The listing builds one solid part. Answer for the finished solid, in the listing's coordinates (mm). A direction names the side the tool comes from. Coordinates: 2 decimals unless noted, no trailing zeros. Order: outer loops, then holes, each group sorted by start corner. A loop starts at its lowest first (then second) coordinate and runs counter-clockwise, first axis right, second up. Notation, with made-up numbers: (69, 48) -> (122, 48) arc R16 cw to (122, 69) -> close; hole circle Ø8 at (35, 17). An arc over 180 degrees is marked (long way). Answer in a Markdown table with one row per item.
```python
from build123d import *

# Parameters (mm, degrees)
RESSALTO_EXTRUS_O1_DEPTH = 55
ESBO_O2_W                = 15.2
ESBO_O2_H                = 25.2
CORTE_EXTRUS_O1_DEPTH    = 3
ESBO_O4_R                = 1.7
CORTE_EXTRUS_O2_DEPTH    = 31
ESBO_O5_R                = 4.7
CORTE_EXTRUS_O3_DEPTH    = 4
ESBO_O6_R                = 1.75
CORTE_EXTRUS_O4_DEPTH    = 4
ESBO_O7_W                = 15
ESBO_O7_H                = 20
ESBO_O7_R                = 1.65
RESSALTO_EXTRUS_O2_DEPTH = 3


with BuildPart() as part:
    # Esboço1 → Ressalto-extrusão1 (new body)
    with BuildSketch(Plane.XY):
        Polygon((0, 0), (38, 0), (38, 8), (3, 8), (3, 30), (0, 30), align=None)
    extrude(amount=RESSALTO_EXTRUS_O1_DEPTH)

    # Esboço2 → Corte-extrusão1 (cut)
    with BuildSketch(Plane.XZ):
        with Locations((28, 30)):
            Rectangle(ESBO_O2_W, ESBO_O2_H)
    extrude(amount=-CORTE_EXTRUS_O1_DEPTH, mode=Mode.SUBTRACT)

    # Esboço4 → Corte-extrusão2 (cut, through all)
    with BuildSketch(Plane.XZ):
        with Locations((28, 30)):
            Circle(ESBO_O4_R)
        with Locations((28, 10)):
            Circle(ESBO_O4_R)
        with BuildLine():
            Line((29.7, 52.5), (29.7, 49.5))
            ThreePointArc((29.7, 49.5), (28, 47.8), (26.3, 49.5))
            Line((26.3, 49.5), (26.3, 52.5))
            ThreePointArc((26.3, 52.5), (28, 54.2), (29.7, 52.5))
        make_face()
    extrude(amount=-CORTE_EXTRUS_O2_DEPTH, mode=Mode.SUBTRACT)

    # Esboço5 → Corte-extrusão3 (cut)
    with BuildSketch(Plane.XZ):
        with Locations((28, 10)):
            Circle(ESBO_O5_R)
        with BuildLine():
            Line((32.7, 49.5), (32.7, 52.5))
            ThreePointArc((32.7, 52.5), (28, 57.2), (23.3, 52.5))
            Line((23.3, 52.5), (23.3, 49.5))
            ThreePointArc((23.3, 49.5), (28, 44.8), (32.7, 49.5))
        make_face()
    extrude(amount=-CORTE_EXTRUS_O3_DEPTH, mode=Mode.SUBTRACT)

    # Esboço6 → Corte-extrusão4 (cut)
    with BuildSketch(Plane.ZY):
        with Locations((48, 20)):
            Circle(ESBO_O6_R)
        with Locations((3, 20)):
            Circle(ESBO_O6_R)
    extrude(amount=-CORTE_EXTRUS_O4_DEPTH, mode=Mode.SUBTRACT)

    # Esboço7 → Ressalto-extrusão2 (add)
    with BuildSketch(Plane.ZY):
        with Locations((62.5, 10)):
            Rectangle(ESBO_O7_W, ESBO_O7_H)
        with Locations((65, 5.25)):
            Circle(ESBO_O7_R, mode=Mode.SUBTRACT)
        with BuildLine():
            Line((63.35, 13.25), (63.35, 16.25))
            ThreePointArc((63.35, 16.25), (65, 17.9), (66.65, 16.25))
            Line((66.65, 16.25), (66.65, 13.25))
            ThreePointArc((66.65, 13.25), (65, 11.6), (63.35, 13.25))
        make_face(mode=Mode.SUBTRACT)
    extrude(amount=-RESSALTO_EXTRUS_O2_DEPTH)


solid = part.part
```
(1) A cutting plane is placed at C-C, the plane z = 65. Determine the outline of the cut face in (x, y), then the cut area to 3 significant figures.
Check values:
| item | result |
|---|---|
| outline | (0, 0) -> (3, 0) -> (3, 3.6) -> (0, 3.6) -> close; (0, 6.9) -> (3, 6.9) -> (3, 11.6) -> (0, 11.6) -> close; (0, 17.9) -> (3, 17.9) -> (3, 20) -> (0, 20) -> close |
| area | 31.2 mm² |
(2) A cutting plane is placed at B-B, the plane z = 3. Determine the outline of the cut face in (x, y).
Check values:
| item | result |
|---|---|
| outline | (0, 0) -> (38, 0) -> (38, 8) -> (3, 8) -> (3, 18.25) -> (0, 18.25) -> close; (0, 21.75) -> (3, 21.75) -> (3, 30) -> (0, 30) -> close |
(3) Find the intervals of material crossed by line 1 along Z through (x, y) = (28, 4.85); line 2 along Y through (x, z) = (2.25, 3); line 3 along X through (y, z) = (3.5, 7.5), in increasing order. Write a range as from..to.
Check values:
| item | result |
|---|---|
| line 1 | 0..8.3, 11.7..28.3, 31.7..47.8, 54.2..55 |
| line 2 | 0..18.25, 21.75..30 |
| line 3 | 0..24.02, 31.98..38 |
(4) A cutting plane is placed at A-A, the plane y = 5.25. Determine the outline of the cut face in (x, z), then the cut area to 3 significant figures.
Check values:
| item | result |
|---|---|
| outline | (0, 0) -> (38, 0) -> (38, 55) -> (3, 55) -> (3, 63.35) -> (0, 63.35) -> close; (0, 66.65) -> (3, 66.65) -> (3, 70) -> (0, 70) -> close; hole circle Ø3.4 at (28, 10); hole circle Ø3.4 at (28, 30); hole (26.3, 49.5) arc R1.7 ccw to (29.7, 49.5) -> (29.7, 52.5) arc R1.7 ccw to (26.3, 52.5) -> close |
| area | 2,090 mm² |
(5) A cutting plane is placed at D-D, the plane x = 22. Determine the outline of the cut face in (y, z), then the cut area to 3 significant figures.
Check values:
| item | result |
|---|---|
| outline | (0, 0) -> (8, 0) -> (8, 55) -> (0, 55) -> (0, 42.6) -> (3, 42.6) -> (3, 17.4) -> (0, 17.4) -> close |
| area | 364 mm² |
(6) Which of the six approach directions +Z, -Z, +X, -X, +Y, -Y give full straight-line access (tool end or side, diameter ignored) to faces 4 (the flat face through (29.7, 6, 51)), 5 (the flat face through (20, 4, 55)), 6 (the cylindrical face through (1.5, 17.9, 65))?
Check values:
| item | result |
|---|---|
| face 4 | +Y, -Y |
| face 5 | +Z, +X, +Y, -Y |
| face 6 | +X, -X |
(7) For a pull along Y with two mould halves and no side action, classify faces 1 (the flat face through (30, 4, 10)), 2 (the flat face through (32.7, 2, 51)), 3 (the flat face through (1, 15, 63.35)) as released by +Y, released by -Y, zero draft, split by the parting line, or undercut.
Check values:
| item | result |
|---|---|
| face 1 | released by -Y |
| face 2 | zero draft |
| face 3 | undercut |
(8) Flat-ended cylindrical pins translate along their axes: pin 1 (2.5 mm diameter, centred on x = 12, y = 5.5, fed in from +Z); pin 2 (4.5 mm diameter, centred on y = 20, z = 3, fed in from +X); pin 3 (1.5 mm diameter, centred on x = 2, z = 64, fed in from +Y); pin 4 (2.5 mm diameter, centred on x = 28, z = 10, fed in from +Y). Find the tip coordinate at first contact, or state that the pin passes through.
Check values:
| item | result |
|---|---|
| pin 1 | z = 55 |
| pin 2 | x = 3 |
| pin 3 | y = 20 |
| pin 4 | through |
